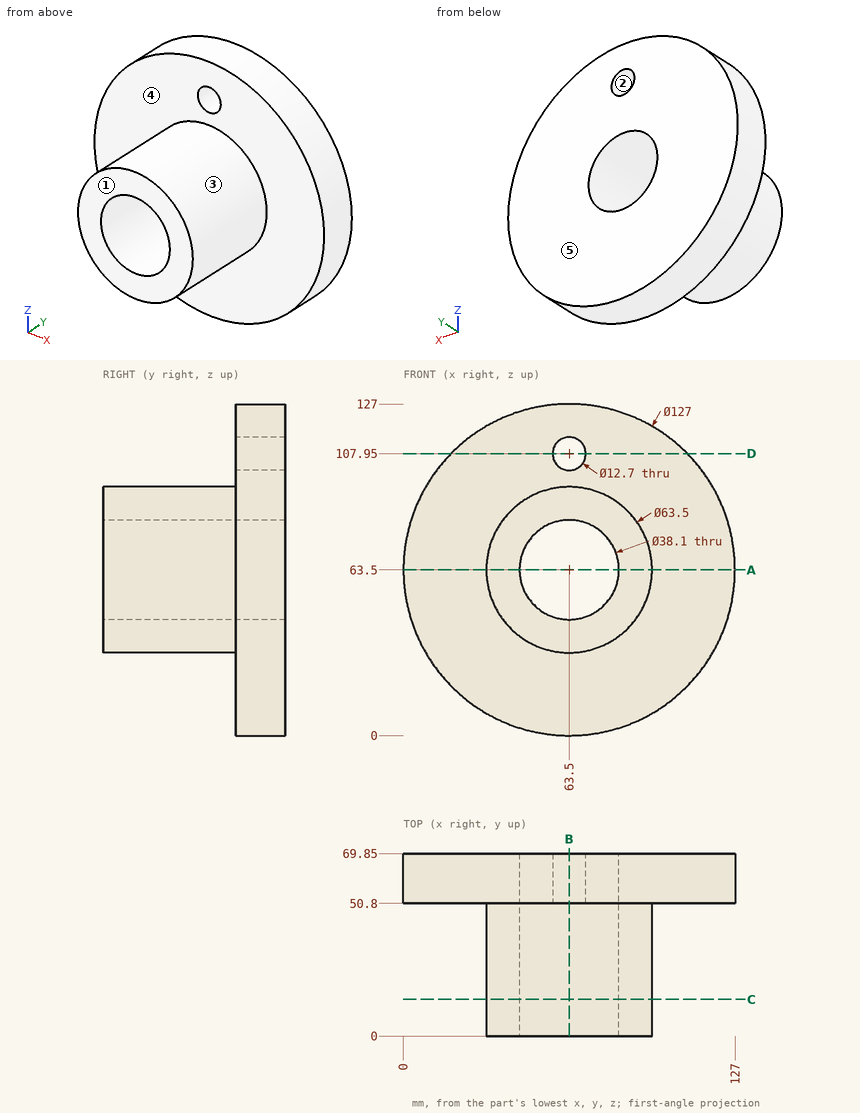
Study the drawing (mm; zero at the part's minimum x, y, z) and answer. A direction names the side the tool comes from. Coordinates: 2 decimals unless noted, no trailing zeros. Loops run counter-clockwise (first coordinate to the right, second up) from the corner with the lowest first, then second, coordinate; pieces in that order, holes last. Notation, with made-up numbers: M 73,-38.75 L 113,-38.75 A33 ccw 113,-3.75 Z; hole C -7.75,35.5 d1. An arc over 180 degrees is marked long. Answer as a JSON object with one key per item and string values. Group by question number.
Item 1: Section D-D (z = 107.95) is taken. Write down the section's boundary in (x, y), and give its area (3 significant figures).
Item 2: Section C-C (y = 14) is taken. Write down the section's boundary in (x, z), and give its area (3 significant figures).
Item 3: Determine the mould class of the marked faces 1, 2 and 3 for opening direction Z: +Z half, -Z half, draft (parallel to the pull), parting line (faces both ways), or undercut.
Item 4: Consider L1, parallel to Z at x = 63, y = 61; L2, parallel to Z at x = 58, y = 53; L3, parallel to Z at x = 63.5, y = 32. Determine where each line is inside the solid, lowest interval first.
Item 5: Which of the six approach directions +Z, -Z, +X, -X, +Y, -Y give full straight-line access (tool end or side, diameter ignored) to the marked faces 4 and 5?
Item 6: Each of these flat-tipped pins is pushed along its axis until it touches: P1, Ø6, axis at y = 59, z = 72, coming from the +X side; P2, Ø12, axis at y = 18, z = 31, coming from the +X side; P3, Ø4, axis at y = 38.5, z = 77, coming from the +X side. Where does it stop, or does it pass through?
Item 7: Section A-A (z = 63.5) is taken. Write down the section's boundary in (x, y).
Item 8: Section B-B (x = 63.5) is taken. Write down the section's boundary in (y, z).
Solved:
{
 "1": {"outline": "M 18.15,50.8 L 57.15,50.8 L 57.15,69.85 L 18.15,69.85 Z; M 69.85,50.8 L 108.85,50.8 L 108.85,69.85 L 69.85,69.85 Z", "area": "1,490 mm2"},
 "2": {"outline": "C 63.5,63.5 d63.5; hole C 63.5,63.5 d38.1", "area": "2,030 mm2"},
 "3": {"face 1": "draft", "face 2": "undercut", "face 3": "parting line"},
 "4": {"L1": "z = 0 to 44.46, 82.54 to 101.62, 114.28 to 127", "L2": "z = 0.24 to 45.26, 81.74 to 104.78, 111.12 to 126.76", "L3": "z = 31.75 to 44.45, 82.55 to 95.25"},
 "5": {"face 4": "-Y", "face 5": "+Z, -Z, +X, -X, +Y"},
 "6": {"P1": "stops at x = 126.76", "P2": "stops at x = 80.99", "P3": "stops at x = 93.09"},
 "7": {"outline": "M 0,50.8 L 31.75,50.8 L 31.75,0 L 44.45,0 L 44.45,69.85 L 0,69.85 Z; M 82.55,0 L 95.25,0 L 95.25,50.8 L 127,50.8 L 127,69.85 L 82.55,69.85 Z"},
 "8": {"outline": "M 0,31.75 L 50.8,31.75 L 50.8,0 L 69.85,0 L 69.85,44.45 L 0,44.45 Z; M 0,82.55 L 69.85,82.55 L 69.85,101.6 L 50.8,101.6 L 50.8,95.25 L 0,95.25 Z; M 50.8,114.3 L 69.85,114.3 L 69.85,127 L 50.8,127 Z"}
}
